Source: CAD feature listing. Evaluate the final solid. Frame: model axes, mm. A direction names the side the tool comes from. Coordinates: 2 decimals unless noted, no trailing zeros. Order: outer loops, then holes, each group sorted by start corner. A loop starts at its lowest first (then second) coordinate and runs counter-clockwise, first axis right, second up.
Item 1: Section A-A on y = 0. Return the cut outline in (x, z).
Item 2: Section C-C on y = 16. Return the cut outline in (x, z).
Item 3: Mould query, pull axis Y, two halves, no side actions, for faces 3 (the cylindrical face through (-5.883, -0.054, 2.465)), 4 (the cylindrical face through (18.76, -32.02, 2.46)), 5 (the flat face through (-0.7, 14.867, 2.465)), 6 (the flat face through (20, 5, 2)). Classes: released by +Y, released by -Y, zero draft, split by the parting line, or undercut.
Item 4: Section D-D on x = -11. Return the cut outline in (y, z).
Item 5: Ray query, line 1 (Y direction, x = -17, z = 4); line 2 (X direction, y = 2, z = 1.75); line 3 (Y direction, x = 20, z = 1.5). Return the intervals inside material, ascending.
Item 6: Reachability of faces 1 (the flat face through (20, -5, 2)), 2 (the cylindrical face through (-10.55, -9.03, 2.46)) from +Z, -Z, +X, -X, +Y, -Y: full face, straight path, thin tool, end or side. Return the list, or none.
Item 7: Contact query for flat-ended pins moving along their axis: P1, Ø4.5, axis at x = 17.7, y = 24.09, coming from the +Z side; P2, Ø2, axis at y = 7.5, z = 2.5, coming from the -X side; P3, Ø3, axis at y = -24.5, z = 4.5, coming from the -X side; P4, Ø1.5, axis at y = 7.5, z = 2.5, coming from the -X side. Output: stop coordinate, or through.
Item 8: Section B-B on z = 2.5. Return the cut outline in (x, y), then the cut area to 3 significant figures.
from build123d import *

# Parameters (mm, degrees)
ESQUISSE1_R        = 1.9
ESQUISSE1_R_2      = 4.4
ESQUISSE1_W        = 4.89999982
ESQUISSE1_H        = 8.00000038
BOSS_EXTRU_1_DEPTH = 5


with BuildPart() as part:
    # Esquisse1 → Boss.-Extru.1 (new body)
    with BuildSketch(Plane.XY):
        with BuildLine():
            Line((25.70156774, 24.190208374), (25.70156774, -24.190208374))
            ThreePointArc((25.70156774, -24.190208374), (18.599090239, -32.039774771), (9.926188952, -25.970041455))
            ThreePointArc((9.926188952, -25.970041455), (8.175930594, -22.028307987), (5.145100617, -18.959963694))
            Line((5.145100617, -18.959963694), (-6.383895202, -10.887273587))
            ThreePointArc((-6.383895202, -10.887273587), (-10.60979376, -9.014950874), (-15.229887052, -8.87875638))
            ThreePointArc((-15.229887052, -8.87875638), (-25.702193121, 0), (-15.229887052, 8.87875638))
            ThreePointArc((-15.229887052, 8.87875638), (-10.60979376, 9.014950873), (-6.383895202, 10.887273587))
            Line((-6.383895202, 10.887273587), (5.145100617, 18.959963694))
            ThreePointArc((5.145100617, 18.959963694), (8.175930651, 22.028307983), (9.926189014, 25.970041482))
            ThreePointArc((9.926189014, 25.970041482), (18.59909026, 32.03977477), (25.70156774, 24.190208374))
        make_face()
        with Locations((17.70219274, 24.090210327)):
            Circle(ESQUISSE1_R, mode=Mode.SUBTRACT)
        with Locations((17.70219274, -24.090210327)):
            Circle(ESQUISSE1_R, mode=Mode.SUBTRACT)
        with Locations((-16.70219312, 0)):
            Circle(ESQUISSE1_R_2, mode=Mode.SUBTRACT)
        with BuildLine():
            Line((8.98146324, -12.490403838), (-4.177200867, -3.276608186))
            ThreePointArc((-4.177200867, -3.276608186), (-5.882895134, 0), (-4.177200867, 3.276608186))
            Line((-4.177200867, 3.276608186), (8.98146324, 12.490403838))
            ThreePointArc((8.98146324, 12.490403838), (12.087438212, 12.693980299), (13.70219255, 10.032948107))
            Line((13.70219255, 10.032948107), (13.70219255, -10.032948107))
            ThreePointArc((13.70219255, -10.032948107), (12.087438212, -12.693980299), (8.98146324, -12.490403838))
        make_face(mode=Mode.SUBTRACT)
        with Locations((19.777192636, 9.000000078)):
            Rectangle(ESQUISSE1_W, ESQUISSE1_H, mode=Mode.SUBTRACT)
        with Locations((19.777192636, -9.000000078)):
            Rectangle(ESQUISSE1_W, ESQUISSE1_H, mode=Mode.SUBTRACT)
    extrude(amount=BOSS_EXTRU_1_DEPTH)


solid = part.part
Answer list:
1. outline: (-25.7, 0) - (-21.1, 0) - (-21.1, 5) - (-25.7, 5) - close; (-12.3, 0) - (-5.88, 0) - (-5.88, 5) - (-12.3, 5) - close; (13.7, 0) - (25.7, 0) - (25.7, 5) - (13.7, 5) - close
2. outline: (0.92, 0) - (25.7, 0) - (25.7, 5) - (0.92, 5) - close
3. face 3: undercut
3. face 4: released by -Y
3. face 5: released by +Y
3. face 6: undercut
4. outline: (-8.93, 0) - (8.93, 0) - (8.93, 5) - (-8.93, 5) - close
5. line 1: y = -9 to -4.39, 4.39 to 9
5. line 2: x = -25.48 to -20.62, -12.78 to -5.35, 13.7 to 25.7
5. line 3: y = -31.75 to -13, -5 to 5, 13 to 31.75
6. face 1: +Z, -Z
6. face 2: +Z, -Z, -Y
7. P1: stops at z = 5
7. P2: stops at x = -22.93
7. P3: stops at x = 8.77
7. P4: stops at x = -22.66
8. outline: (-15.23, -8.88) arc R12 cw to (-6.38, -10.89) - (5.15, -18.96) arc R12 cw to (9.93, -25.97) arc R8 ccw to (25.7, -24.19) - (25.7, 24.19) arc R8 ccw to (9.93, 25.97) arc R12 cw to (5.15, 18.96) - (-6.38, 10.89) arc R12 cw to (-15.23, 8.88) arc R9 ccw (long way) to start; hole circle Ø8.8 at (-16.7, 0); hole (-4.18, -3.28) - (8.98, -12.49) arc R3 ccw to (13.7, -10.03) - (13.7, 10.03) arc R3 ccw to (8.98, 12.49) - (-4.18, 3.28) arc R4 ccw to start; hole circle Ø3.8 at (17.7, -24.09); hole circle Ø3.8 at (17.7, 24.09); hole (17.33, -13) - (22.23, -13) - (22.23, -5) - (17.33, -5) - close; hole (17.33, 5) - (22.23, 5) - (22.23, 13) - (17.33, 13) - close
8. area: 1,330 mm2
